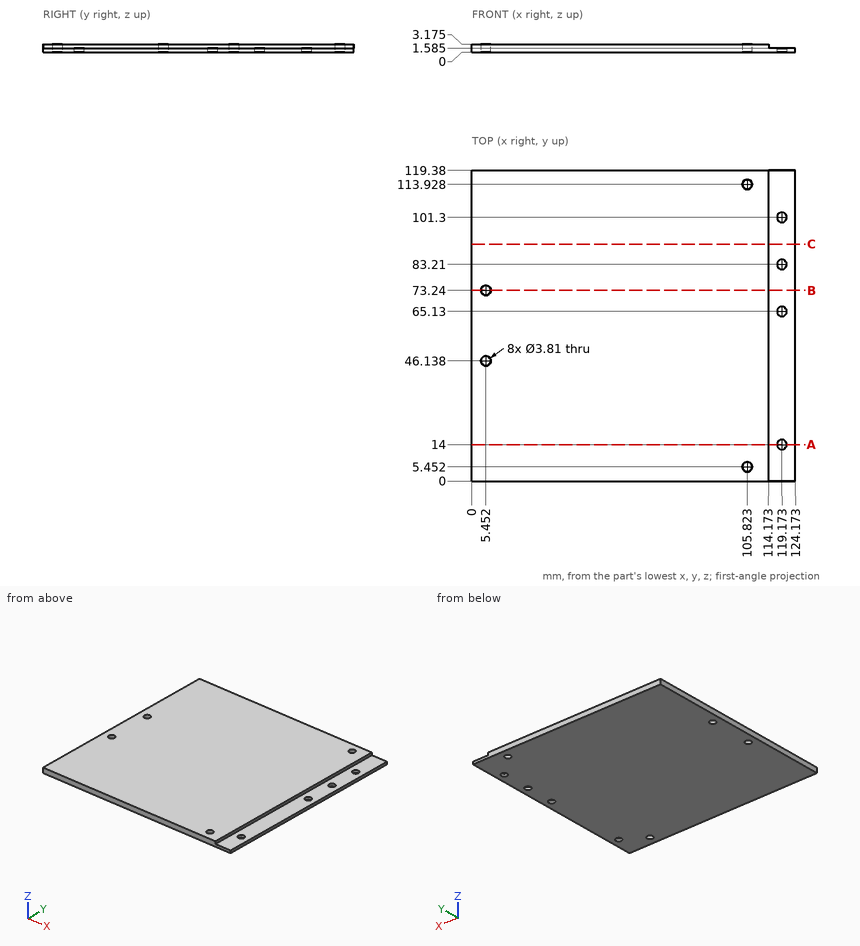
Can you work these out from the drawing? Everything is in mm from the part's minimum corner. Round coordinates to 2 decimals unless told otherwise and drop trailing zeros. Loops run counter-clockwise (first coordinate to the right, second up) from the corner with the lowest first, then second, coordinate; pieces in that order, holes last.
1. If we section it at A-A on y = 14: Write out the boundary of the cut face in (x, z) (3 decimals), plus the area to 3 significant figures.
Answer list:
outline: (0, 0) - (117.268, 0) - (117.268, 1.585) - (114.173, 1.585) - (114.173, 3.175) - (0, 3.175) - close; (121.078, 0) - (124.173, 0) - (124.173, 1.585) - (121.078, 1.585) - close
area: 372 mm2
2. If I drill on line 1 along Y through (x, z) = (106.5, 2.4); line 2 along Z through (x, y) = (117, 10) (3 decimals); line 3 along X through (y, z) = (35, 2.05), over which ranges is the centre line in solid material (lowest first)?
Answer list:
line 1: y = 0 to 3.67, 7.23 to 112.15, 115.71 to 119.38
line 2: z = 0 to 1.585
line 3: x = 0 to 114.17
3. If we section it at B-B on y = 73.24: Write out the boundary of the cut face in (x, z) (3 decimals).
Answer list:
outline: (0, 0) - (3.547, 0) - (3.547, 3.175) - (0, 3.175) - close; (7.357, 0) - (124.173, 0) - (124.173, 1.585) - (114.173, 1.585) - (114.173, 3.175) - (7.357, 3.175) - close
4. If we section it at C-C on y = 91: Write out the boundary of the cut face in (x, z) (3 decimals).
Answer list:
outline: (0, 0) - (124.173, 0) - (124.173, 1.585) - (114.173, 1.585) - (114.173, 3.175) - (0, 3.175) - close
5. For P1, Ø6, axis at x = 119.173, y = 83.21, coming from the +Z side (3 decimals); P2, Ø2.5, axis at x = 119.173, y = 65.13, coming from the -Z side; P3, Ø5, axis at x = 119.173, y = 14, coming from the -Z side, each with a flat end and sliding along its axis, tell me the tip position at first contact or that it passes through.
Answer list:
P1: stops at z = 1.585
P2: passes through
P3: stops at z = 0
